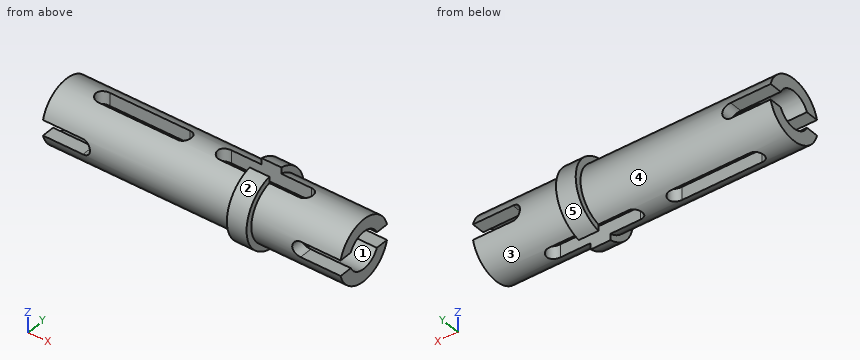
```python
from build123d import *

# Parameters (mm, degrees)
SKETCH1_R                = 3
BOSS_EXTRUDE1_DEPTH      = 0.8
BOSS_EXTRUDE2_DEPTH      = 7.2
BOSS_EXTRUDE2_DEPTH_BACK = 17
SKETCH2_R                = 2.5
CUT_EXTRUDE1_DEPTH       = 17.746342884
CUT_EXTRUDE1_DEPTH_BACK  = 17.746342884
SKETCH4_R                = 1.5
CUT_EXTRUDE2_DEPTH       = 25.561135557
CUT_EXTRUDE3_DEPTH       = 17.734675923
CUT_EXTRUDE3_DEPTH_BACK  = 17.734675923


with BuildPart() as part:
    # Sketch1 → Boss-Extrude1 (new, symmetric)
    with BuildSketch(Plane(origin=(0, 0, 0), x_dir=(0, 0, -1), z_dir=(1, 0, 0))):
        Circle(SKETCH1_R)
    extrude(amount=BOSS_EXTRUDE1_DEPTH, both=True)

    # Sketch2 → Boss-Extrude2 (add, two sides: drawn at the far end of the back side and taken through both)
    with BuildSketch(Plane(origin=(0.8, 0, 0), x_dir=(0, 0, -1), z_dir=(1, 0, 0)).offset(-BOSS_EXTRUDE2_DEPTH_BACK)):
        Circle(SKETCH2_R)
    extrude(amount=BOSS_EXTRUDE2_DEPTH + BOSS_EXTRUDE2_DEPTH_BACK)

    # Sketch3 → Cut-Extrude1 (cut, two sides: drawn at the far end of the back side and taken through both)
    with BuildSketch(Plane.XY.offset(-CUT_EXTRUDE1_DEPTH_BACK)):
        with BuildLine():
            Line((-3.25, 0.625), (3.25, 0.625))
            ThreePointArc((3.25, 0.625), (3.875, 0), (3.25, -0.625))
            Line((3.25, -0.625), (-3.25, -0.625))
            ThreePointArc((-3.25, -0.625), (-3.875, 0), (-3.25, 0.625))
        make_face()
        with BuildLine():
            Line((-13.139009245, 0.625), (-6.639009245, 0.625))
            ThreePointArc((-6.639009245, 0.625), (-6.014009245, 0), (-6.639009245, -0.625))
            Line((-6.639009245, -0.625), (-13.139009245, -0.625))
            ThreePointArc((-13.139009245, -0.625), (-13.764009245, 0), (-13.139009245, 0.625))
        make_face()
    extrude(amount=CUT_EXTRUDE1_DEPTH + CUT_EXTRUDE1_DEPTH_BACK, mode=Mode.SUBTRACT)

    # Sketch4 → Cut-Extrude2 (cut, through all)
    with BuildSketch(Plane(origin=(8, 0, 0), x_dir=(0, 0, -1), z_dir=(1, 0, 0))):
        Circle(SKETCH4_R)
    extrude(amount=-CUT_EXTRUDE2_DEPTH, mode=Mode.SUBTRACT)

    # Sketch5 → Cut-Extrude3 (cut, two sides: drawn at the far end of the back side and taken through both)
    with BuildSketch(Plane(origin=(0, 0, 0), x_dir=(1, 0, 0), z_dir=(0, 1, 0)).offset(-CUT_EXTRUDE3_DEPTH_BACK)):
        with BuildLine():
            Line((-19.45, 0.625), (-12.95, 0.625))
            ThreePointArc((-12.95, 0.625), (-12.325, 0), (-12.95, -0.625))
            Line((-12.95, -0.625), (-19.45, -0.625))
            ThreePointArc((-19.45, -0.625), (-20.075, 0), (-19.45, 0.625))
        make_face()
        with BuildLine():
            Line((11.25, -0.625), (4.75, -0.625))
            ThreePointArc((4.75, -0.625), (4.125, 0), (4.75, 0.625))
            Line((4.75, 0.625), (11.25, 0.625))
            ThreePointArc((11.25, 0.625), (11.875, 0), (11.25, -0.625))
        make_face()
    extrude(amount=CUT_EXTRUDE3_DEPTH + CUT_EXTRUDE3_DEPTH_BACK, mode=Mode.SUBTRACT)


solid = part.part
```
Design review of the part built by this model. Coordinates are the model's own, in mm. Face numbers are marked on the shaded views. A direction names the side the tool comes from. Coordinates: 2 decimals unless noted, no trailing zeros. Order: outer loops, then holes, each group sorted by start corner. A loop starts at its lowest first (then second) coordinate and runs counter-clockwise, first axis right, second up.
1) Take a section at A-A, the plane y = 0. Give the boundary of the cut face in (x, z) (3 decimals).
2) For the marked faces 3, 4 and 5, list the 3-axis set-ups (+Z, -Z, +X, -X, +Y, -Y) from which the entire face can be reached by the end or side of a thin tool; tool diameter is ignored.
3) Clearance check with flat-ended pins moving along their axes: pin 1 (1.2 mm diameter, centred on x = 6, y = 1.5, fed in from -Z); pin 2 (0.5 mm diameter, centred on x = -9.5, z = 2, fed in from +Y); pin 3 (0.5 mm diameter, centred on x = -14.5, y = -2, fed in from -Z). State where each tip first meets the part, or that it passes through.
4) Take a section at D-D, the plane x = -3.5. Give the boundary of the cut face in (y, z), and give its area (3 significant figures).
5) Mouldability with a two-part tool opening along Z and no side actions: class the marked faces 1 and 2 as +Z half, -Z half, draft (parallel to the pull), parting line (faces both ways), or undercut.
6) Wall thickness on line 1 along X through (y, z) = (0, 2.1) (3 decimals); line 2 along Y through (x, z) = (-3, 0): over which ranges is each line inside the solid? List them lowest first.
7) Take a section at C-C, the plane z = 0. Give the boundary of the cut face in (x, y) (3 decimals).
8) Take a section at B-B, the plane x = -0.5. Give the boundary of the cut face in (y, z) (3 decimals).
Returned:
1. outline: (-16.2, -2.5) - (-13.764, -2.5) - (-13.764, -1.5) - (-16.2, -1.5) - close; (-16.2, 1.5) - (-13.764, 1.5) - (-13.764, 2.5) - (-16.2, 2.5) - close; (-6.014, -2.5) - (-3.875, -2.5) - (-3.875, -1.5) - (-6.014, -1.5) - close; (-6.014, 1.5) - (-3.875, 1.5) - (-3.875, 2.5) - (-6.014, 2.5) - close; (3.875, -2.5) - (8, -2.5) - (8, -1.5) - (3.875, -1.5) - close; (3.875, 1.5) - (8, 1.5) - (8, 2.5) - (3.875, 2.5) - close
2. face 3: +X
2. face 4: -X
2. face 5: +X, -X, +Y
3. pin 1: stops at z = -2.33
3. pin 2: stops at y = 1.79
3. pin 3: stops at z = -1.79
4. outline: (-0.57, -2.43) - (-0.57, -1.39) arc R1.5 cw to (-0.57, 1.39) - (-0.57, 2.43) arc R2.5 ccw to start; (0.57, -2.43) arc R2.5 ccw to (0.57, 2.43) - (0.57, 1.39) arc R1.5 cw to (0.57, -1.39) - close
4. area: 10.2 mm2
5. face 1: undercut
5. face 2: parting line
6. line 1: x = -16.2 to -13.764, -6.014 to -3.875, 3.875 to 8
6. line 2: y = -2.5 to -1.5, 1.5 to 2.5
7. outline: (-12.325, -2.5) - (-0.8, -2.5) - (-0.8, -3) - (0.8, -3) - (0.8, -2.5) - (4.125, -2.5) - (4.125, -1.5) - (-12.325, -1.5) - close; (-12.325, 1.5) - (4.125, 1.5) - (4.125, 2.5) - (0.8, 2.5) - (0.8, 3) - (-0.8, 3) - (-0.8, 2.5) - (-12.325, 2.5) - close
8. outline: (-0.625, -2.934) - (-0.625, -1.364) arc R1.5 cw to (-0.625, 1.364) - (-0.625, 2.934) arc R3 ccw to start; (0.625, -2.934) arc R3 ccw to (0.625, 2.934) - (0.625, 1.364) arc R1.5 cw to (0.625, -1.364) - close
